For this review, take the finished solid that the model builds, in its own axes (mm). A direction names the side the tool comes from. Coordinates: 2 decimals unless noted, no trailing zeros. Write each loop counter-clockwise with the first axis right and the second up, starting at its lowest first coordinate (ties: lowest second). Pieces come first, ordered by that corner, then holes.
```python
from build123d import *

# Parameters (mm, degrees)
BOSS_EXTRUDE1_DEPTH = 1
BOSS_EXTRUDE2_DEPTH = 12
SKETCH2_W           = 10
SKETCH2_H           = 11
SKETCH2_W_2         = 12
CUT_EXTRUDE1_DEPTH  = 12
SKETCH3_R           = 2.5
CUT_EXTRUDE2_DEPTH  = 12


with BuildPart() as part:
    # Sketch1 → Boss-Extrude1 (new body)
    with BuildSketch(Plane(origin=(0, 0, 0), x_dir=(1, 0, 0), z_dir=(0, 1, 0))):
        Polygon((-1.2, 1.2), (44.2, 1.2), (44.2, -65.8), (65.2, -65.8), (65.2, -123.2), (36.2, -123.2), (36.2, -168.2), (-1.2, -168.2), align=None)
        Polygon((0, -167), (35, -167), (35, -122), (64, -122), (64, -67), (43, -67), (43, 0), (0, 0), align=None, mode=Mode.SUBTRACT)
        Polygon((0, 0), (0, -167), (35, -167), (35, -122), (64, -122), (64, -67), (43, -67), (43, 0), align=None)
    extrude(amount=BOSS_EXTRUDE1_DEPTH)

    # Sketch1<3> → Boss-Extrude2 (add)
    with BuildSketch(Plane(origin=(0, 0, 0), x_dir=(1, 0, 0), z_dir=(0, 1, 0))):
        Polygon((-1.2, 1.2), (-1.2, -168.2), (36.2, -168.2), (36.2, -123.2), (65.2, -123.2), (65.2, -65.8), (44.2, -65.8), (44.2, 1.2), align=None)
        Polygon((0, 0), (0, -167), (35, -167), (35, -122), (64, -122), (64, -67), (43, -67), (43, 0), align=None, mode=Mode.SUBTRACT)
    extrude(amount=BOSS_EXTRUDE2_DEPTH)

    # Sketch2 → Cut-Extrude1 (cut)
    with BuildSketch(Plane(origin=(65.2, 0, 0), x_dir=(0, 0, -1), z_dir=(1, 0, 0))):
        with Locations((-72.8, 6.5)):
            Rectangle(SKETCH2_W, SKETCH2_H)
        with Locations((-107.2, 6.5)):
            Rectangle(SKETCH2_W_2, SKETCH2_H)
    extrude(amount=-CUT_EXTRUDE1_DEPTH, mode=Mode.SUBTRACT)

    # Sketch3 → Cut-Extrude2 (cut)
    with BuildSketch(Plane(origin=(0, 1, 0), x_dir=(1, 0, 0), z_dir=(0, 1, 0))):
        with Locations(Location((5.592629817, -7.1408635, 0), (0, 0, 270))):
            Circle(SKETCH3_R)
        with Locations(Location((20.139491033, -7.350170855, 0), (0, 0, 270))):
            Circle(SKETCH3_R)
        with Locations(Location((32.488625014, -7.036209822, 0), (0, 0, 270))):
            Circle(SKETCH3_R)
        with Locations(Location((7.999664407, -59.67700976, 0), (0, 0, 270))):
            Circle(SKETCH3_R)
        with Locations(Location((34.895659604, -59.572356082, 0), (0, 0, 270))):
            Circle(SKETCH3_R)
        with Locations(Location((9.579399834, -108.003673304, 0), (0, 0, 270))):
            Circle(SKETCH3_R)
        with Locations(Location((36.475395031, -107.899019626, 0), (0, 0, 270))):
            Circle(SKETCH3_R)
        with Locations(Location((4.511546122, -160.279750326, 0), (0, 0, 270))):
            Circle(SKETCH3_R)
        with Locations(Location((31.407541319, -160.175096649, 0), (0, 0, 270))):
            Circle(SKETCH3_R)
    extrude(amount=-CUT_EXTRUDE2_DEPTH, mode=Mode.SUBTRACT)


solid = part.part
```
1) Tool access review of faces 1 (the face through (25, 0, 82)), 2 (the face through (35, 6, 145)), 3 (the face through (36.2, 6, 145)): name each direction out of +Z, -Z, +X, -X, +Y, -Y from which nothing blocks a thin tool from reaching the whole face with its end or side.
2) Consider section B-B (x = 14). Give the boundary of the cut face in (y, z).
3) The part is to be moulded in two halves that separate along Z. For faces 4 (the face through (18, 6, 168.2)), 5 (the face through (44.2, 6, 32)), 6 (the face through (4.07, 0.51, 5.16)), say which applies: pulls with the +Z half, pulls with the -Z half, needs draft (parallel to the pull), parting line crosses it, or undercut.
4) Clearance check with flat-ended pins moving along their axes: P1, Ø1.3, axis at x = 64.5, y = 6.5, coming from the +Z side; P2, Ø1, axis at x = 6.5, z = 25.5, coming from the +Y side; P3, Ø3.5, axis at y = 3.5, z = 25, coming from the +X side. State where each tip first meets the part, or that it passes through.
5) Consider section C-C (z = 35.5). Give the boundary of the cut face in (x, y), then the cut area to 3 significant figures.
6) Consider section D-D (z = 108). Give the boundary of the cut face in (x, y).
7) For L1, parallel to Z at x = 50, y = 3.75; L2, parallel to Z at x = 38, y = 4.75; L3, parallel to X at y = 3, z = 88, list the stretches that pass through material, from the lowest coordinate up.
8) Consider section A-A (y = 6.5). Give the boundary of the cut face in (x, z), then the cut area to 3 significant figures.
Results:
1. face 1: +Z, -Z, +X, -X, -Y
1. face 2: +Y
1. face 3: +Z, +X, +Y, -Y
2. outline: (0, -1.2) - (12, -1.2) - (12, 0) - (1, 0) - (1, 167) - (12, 167) - (12, 168.2) - (0, 168.2) - close
3. face 4: pulls with the +Z half
3. face 5: needs draft
3. face 6: undercut
4. P1: stops at z = 123.2
4. P2: stops at y = 1
4. P3: stops at x = 44.2
5. outline: (-1.2, 0) - (44.2, 0) - (44.2, 12) - (43, 12) - (43, 1) - (0, 1) - (0, 12) - (-1.2, 12) - close
5. area: 71.8 mm2
6. outline: (-1.2, 0) - (7.08, 0) - (7.08, 1) - (0, 1) - (0, 12) - (-1.2, 12) - close; (12.08, 0) - (33.98, 0) - (33.98, 1) - (12.08, 1) - close; (38.97, 0) - (65.2, 0) - (65.2, 1) - (38.97, 1) - close
7. L1: z = 65.8 to 67, 122 to 123.2
7. L2: z = -1.2 to 0, 122 to 123.2
7. L3: x = -1.2 to 0, 64 to 65.2
8. outline: (-1.2, -1.2) - (44.2, -1.2) - (44.2, 65.8) - (65.2, 65.8) - (65.2, 67.8) - (64, 67.8) - (64, 67) - (43, 67) - (43, 0) - (0, 0) - (0, 167) - (35, 167) - (35, 122) - (64, 122) - (64, 113.2) - (65.2, 113.2) - (65.2, 123.2) - (36.2, 123.2) - (36.2, 168.2) - (-1.2, 168.2) - close; (64, 77.8) - (65.2, 77.8) - (65.2, 101.2) - (64, 101.2) - close
8. area: 534 mm2
